from build123d import *

# Parameters (mm, degrees)
F0_R      = 12.7
F1_DEPTH  = 30.1625
F3_DEPTH  = 19.05
F4_W      = 32.8422
F4_H      = 22.352
F5_DEPTH  = 19.05
F6_R      = 6.35
F7_DEPTH  = 22.353
F9_W      = 44.704
F9_H      = 22.3266
F10_DEPTH = 149.353


with BuildPart() as f1:
    # F0 (on Front) → F1 (new body, symmetric)
    with BuildSketch(Plane.XZ):
        with BuildLine():
            Line((194.2084, 0), (22.352, 0))
            ThreePointArc((22.352, 0), (-15.805251, 15.805251), (0, -22.352))
            Line((0, -22.352), (194.2084, -22.352))
            Line((194.2084, -22.352), (194.2084, 0))
        make_face()
        Circle(F0_R, mode=Mode.SUBTRACT)
    extrude(amount=F1_DEPTH, both=True)

    # F2 (on face) → F3 (cut)
    with BuildSketch(Plane.XZ.offset(30.1625)):
        Polygon((91.8464, -22.352), (150.0886, -22.352), (150.0886, 0), (85.852, 0), align=None)
    extrude(amount=-F3_DEPTH, mode=Mode.SUBTRACT)

    # F4 (on face) → F5 (join)
    with BuildSketch(Plane.XZ.offset(11.1125)):
        with BuildLine():
            Line((117.2464, 0), (150.0886, 0))
            Line((150.0886, 0), (150.0886, 29.718))
            ThreePointArc((150.0886, 29.718), (148.600702, 33.310102), (145.0086, 34.798))
            Line((145.0086, 34.798), (131.0386, 34.798))
            ThreePointArc((131.0386, 34.798), (127.464415, 16.082358), (117.2464, 0))
        make_face()
        with Locations((133.6675, -11.176)):
            Rectangle(F4_W, F4_H)
    extrude(amount=F5_DEPTH)

    # F6 (on Top) → F7 (cut, through all)
    with BuildSketch(Plane.XY):
        with Locations((155.3464, 7.8105)):
            Circle(F6_R)
    extrude(amount=-F7_DEPTH, mode=Mode.SUBTRACT)

    # F9 (on offset) → F10 (cut, through all)
    with BuildSketch(Plane.XY.offset(127)):
        Rectangle(F9_W, F9_H)
    extrude(amount=-F10_DEPTH, mode=Mode.SUBTRACT)


solid = f1.part
CAD build for the part. Positions are in the model's coordinates, mm. A direction names the side the tool comes from. Coordinates: 2 decimals unless noted, no trailing zeros. Write each loop counter-clockwise with the first axis right and the second up, starting at its lowest first coordinate (ties: lowest second). Pieces come first, ordered by that corner, then holes. Notation, with made-up numbers: (-2, 66) - (40, 66) arc R17 ccw to (40, 77) - close; hole circle Ø7 at (37.5, -40). An arc over 180 degrees is marked (long way). Use a Markdown table: item, result. Add a question column.
Item 1: Band-saw the part on D-D, the plane x = 136. Give the cut face in (y, z), and give its area (3 significant figures).
Item 2: Band-saw the part on B-B, the plane y = 17. Give the cut face in (x, z).
Item 3: Drill centre lines: L1, parallel to Z at x = 0, y = 24; L2, parallel to X at y = -13.5, z = -10.5; L3, parallel to Z at x = 33, y = -23. Where is each one in solid material? Low to high. Write a range as from..to.
Item 4: Mould opens along Z. For faces 4 (the face through (34, -30.162, -5)), 5 (the face through (-2.75, 20.8, -12.4)), 6 (the face through (-15.275, 20.53, 16.318)) say: pulls with the +Z half, pulls with the -Z half, needs draft (parallel to the pull), parting line crosses it, or undercut.
Item 5: Band-saw the part on C-C, the plane x = 6.5. Give the cut face in (y, z).
Item 6: Band-saw the part on A-A, the plane y = -24. Give the cut face in (x, z).
Item 7: Flat gauge pins, fed straight in: pin 1 (16.5 mm diameter, centred on x = 135, z = 21.5, fed in from +Y); pin 2 (8 mm diameter, centred on y = -18, z = 14.5, fed in from -X); pin 3 (21 mm diameter, centred on y = -21.5, z = -15.5, fed in from -X); pin 4 (13.5 mm diameter, centred on x = -3, z = 1.5, fed in from +Y). Where does each tip first touch, or does it go through?
Item 8: 3-axis set-ups, long thin cutter, end or side, ignore diameter. For faces 1 (the face through (88.8, -20.8, -11)), 2 (the face through (137, -11.112, 18)), 3 (the face through (127.56, -20.5, 16.33)): which of +Z, -Z, +X, -X, +Y, -Y reach the whole face in a straight line?
Numbers:
| question | item | result |
|---|---|---|
| 1 | outline | (-30.16, -22.35) - (30.16, -22.35) - (30.16, 0) - (-11.11, 0) - (-11.11, 34.8) - (-30.16, 34.8) - close |
| 1 | area | 2,010 mm2 |
| 2 | outline | (0, -22.35) - (194.21, -22.35) - (194.21, 0) - (22.35, 0) arc R22.35 ccw (long way) to start; hole circle Ø25.4 at (0, 0) |
| 3 | L1 | -22.35..-12.7, 12.7..22.35 |
| 3 | L2 | -19.73..-7.14, 7.14..88.67, 117.25..194.21 |
| 3 | L3 | -22.35..0 |
| 4 | face 4 | needs draft |
| 4 | face 5 | undercut |
| 4 | face 6 | parting line crosses it |
| 5 | outline | (-30.16, -22.35) - (-11.16, -22.35) - (-11.16, -10.91) - (-30.16, -10.91) - close; (-30.16, 10.91) - (-11.16, 10.91) - (-11.16, 21.39) - (-30.16, 21.39) - close; (11.16, -22.35) - (30.16, -22.35) - (30.16, -10.91) - (11.16, -10.91) - close; (11.16, 10.91) - (30.16, 10.91) - (30.16, 21.39) - (11.16, 21.39) - close |
| 6 | outline | (0, -22.35) - (91.85, -22.35) - (85.85, 0) - (22.35, 0) arc R22.35 ccw (long way) to start; (117.25, -22.35) - (194.21, -22.35) - (194.21, 0) - (150.09, 0) - (150.09, 29.72) arc R5.08 ccw to (145.01, 34.8) - (131.04, 34.8) arc R50.8 cw to (117.25, 0) - close; hole circle Ø25.4 at (0, 0) |
| 7 | pin 1 | y = -11.11 |
| 7 | pin 2 | x = -19.73 |
| 7 | pin 3 | x = -21.79 |
| 7 | pin 4 | through |
| 8 | face 1 | +Z, -Y |
| 8 | face 2 | +Z, +X, -X, +Y |
| 8 | face 3 | +Z, +Y, -Y |
